Input: dimensioned drawing with shaded views. Units: mm. Origin: part minimum x, y, z. A direction names the side the tool comes from. Give positions to 0.01 mm unless a question says otherwise; leave off trailing zeros. Write each loop counter-clockwise with the first axis right and the second up, starting at its lowest first coordinate (ties: lowest second). Pieces come first, ordered by that corner, then holes. Notation, with made-up numbers: (-32.75, -33.5) -> (24.25, -33.5) arc R3 cw to (24.25, -29.5) -> close; hole circle Ø3 at (87.25, 57). An arc over 180 degrees is marked (long way). Return JSON: item names as keys, results as strings. Group by question number.
Item 1: Section B-B, the plane x = 6.25. Return loops of the section in (y, z), then the cut area to 3 significant figures.
Item 2: Pin query (flat end, axial travel): P1, Ø10, axis at x = 33, y = 8.5, coming from the -Z side; P2, Ø3.5, axis at x = 93.75, z = 40, coming from the +Y side; P3, Ø9.5, axis at x = 93.75, z = 10, coming from the +Y side; P4, Ø1.5, axis at y = 10.5, z = 31, coming from the -X side. Return the tip coordinate at first contact, or that it passes through.
Item 3: Section D-D, the plane z = 10. Return loops of the section in (x, y), then the cut area to 3 significant figures.
Item 4: Section C-C, the plane y = 11.5. Return loops of the section in (x, z), then the cut area to 3 significant figures.
Item 5: Set-up query: the marked faces 1, 2, 3, 4 and 5. Return all of +Z, -Z, +X, -X, +Y, -Y with unobstructed straight access to the full face (end or side cutting, diameter ignored); none if empty.
Item 6: Section A-A, the plane y = 3. Return loops of the section in (x, z), then the cut area to 3 significant figures.
Item 7: Line query: line 1 (X direction, y = 22.75, z = 20); line 2 (X direction, y = 3.75, z = 10); line 3 (Z direction, x = 74.75, y = 21). Output: solid intervals per line, ascending. Write a range as [from, to].
Item 8: Mould query, pull axis X, two halves, no side actions, for the marked faces 6, 7, 8 and 9. Classes: released by +X, released by -X, zero draft, split by the parting line, or undercut.
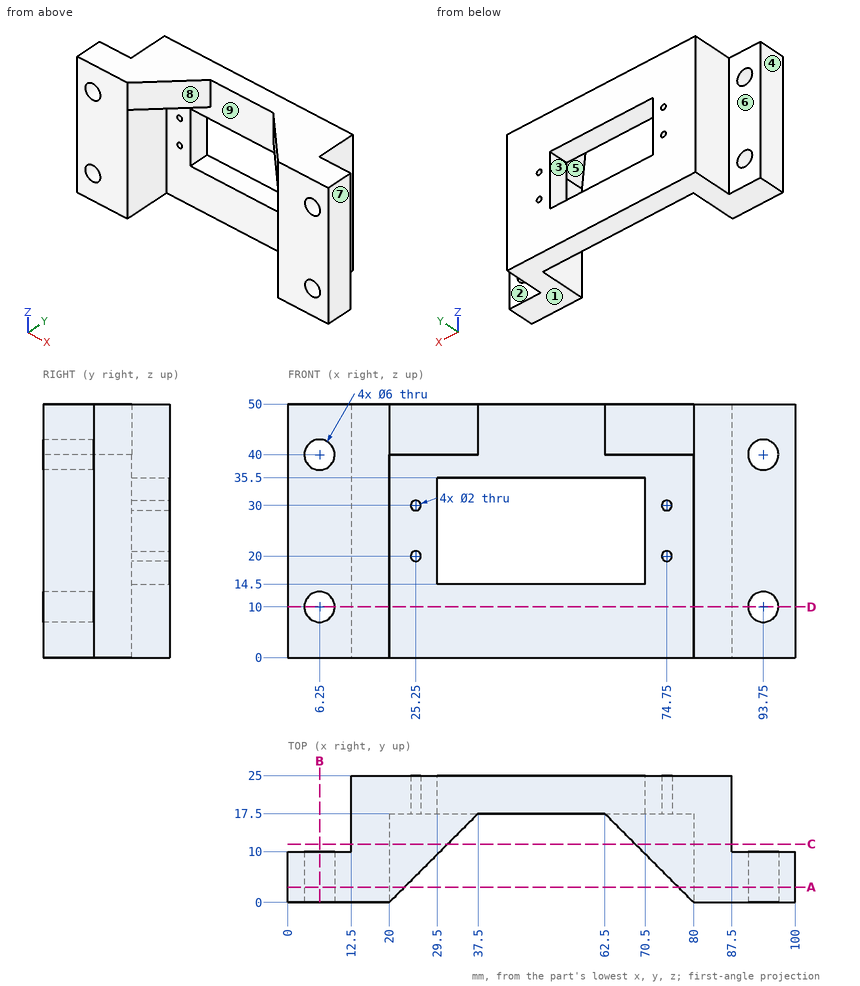
Answer below:
{
 "1": {"outline": "(0, 0) -> (10, 0) -> (10, 7) -> (0, 7) -> close; (0, 13) -> (10, 13) -> (10, 37) -> (0, 37) -> close; (0, 43) -> (10, 43) -> (10, 50) -> (0, 50) -> close", "area": "380 mm2"},
 "2": {"P1": "stops at z = 40", "P2": "passes through", "P3": "stops at y = 10", "P4": "stops at x = 0"},
 "3": {"outline": "(0, 0) -> (3.25, 0) -> (3.25, 10) -> (0, 10) -> close; (9.25, 0) -> (20, 0) -> (20, 17.5) -> (80, 17.5) -> (80, 0) -> (90.75, 0) -> (90.75, 10) -> (87.5, 10) -> (87.5, 25) -> (12.5, 25) -> (12.5, 10) -> (9.25, 10) -> close; (96.75, 0) -> (100, 0) -> (100, 10) -> (96.75, 10) -> close", "area": "955 mm2"},
 "4": {"outline": "(12.5, 0) -> (20, 0) -> (20, 40) -> (31.5, 40) -> (31.5, 50) -> (12.5, 50) -> close; (68.5, 40) -> (80, 40) -> (80, 0) -> (87.5, 0) -> (87.5, 50) -> (68.5, 50) -> close", "area": "980 mm2"},
 "5": {"face 1": "-Z, +X, -X, +Y, -Y", "face 2": "+Z, -Z, +X, +Y", "face 3": "+Y, -Y", "face 4": "+Z, -Z, -X, +Y, -Y", "face 5": "-Z, -Y"},
 "6": {"outline": "(0, 0) -> (20, 0) -> (20, 40) -> (23, 40) -> (23, 50) -> (0, 50) -> close; (77, 40) -> (80, 40) -> (80, 0) -> (100, 0) -> (100, 50) -> (77, 50) -> close; hole circle Ø6 at (6.25, 10); hole circle Ø6 at (6.25, 40); hole circle Ø6 at (93.75, 10); hole circle Ø6 at (93.75, 40)", "area": "1,950 mm2"},
 "7": {"line 1": "x = [12.5, 24.25], [26.25, 29.5], [70.5, 73.75], [75.75, 87.5]", "line 2": "x = [0, 3.25], [9.25, 20], [80, 90.75], [96.75, 100]", "line 3": "z = [0, 19], [21, 29], [31, 50]"},
 "8": {"face 6": "zero draft", "face 7": "released by +X", "face 8": "undercut", "face 9": "undercut"}
}
